Design review of the part built by this model. Coordinates are the model's own, in mm. Coordinates: 2 decimals unless noted, no trailing zeros. Loops run counter-clockwise (first coordinate to the right, second up) from the corner with the lowest first, then second, coordinate; pieces in that order, holes last. Notation, with made-up numbers: (-9, -15) - (39, -15) arc R25 ccw to (39, 4) - close; hole circle Ø9 at (-2, 6.5). An arc over 180 degrees is marked (long way). Use one line per item in the form item = value. Start each with the question number.
(1) Add section B-B (z = -54). State the section outline as (x, y) points.
(2) Add section A-A (z = -32.4). State the section outline as (x, y) points, plus the area to 3 significant figures.
(3) Clearance check with flat-ended pins moving along their axes: pin 1 Ø4.5 at (x, z) = (78.07, -32.4) entering from -Y; pin 2 Ø12.5 at (x, z) = (10, -10) entering from -Y. State where each tip first meets the part, or that it passes through.
(4) For L1, parallel to X at y = 2.75, z = -32.4; L2, parallel to Z at x = 140.5, y = 4.75; L3, parallel to X at y = 3, z = -10, list the stretches that pass through material, from the lowest coordinate up.
(5) Add section C-C (y = 2.25). Count the separate pieces of the cut face and the enclosed holes in it, plus the area to 3 significant figures.
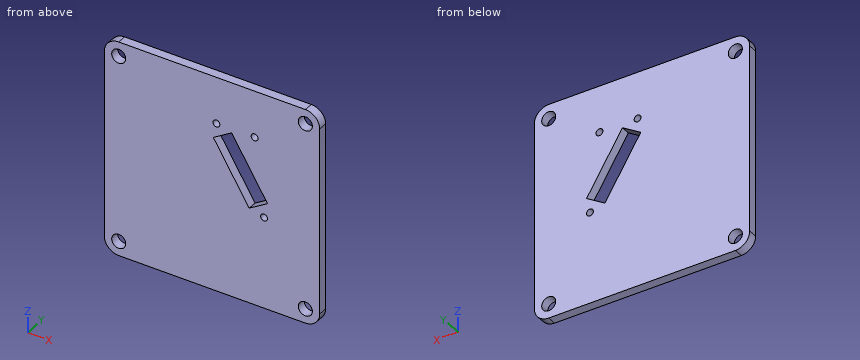
```python
from build123d import *

# Parameters (mm, degrees)
BOSS_EXTRUDE1_DEPTH = 6.35
SKETCH2_R           = 2.4
SKETCH2_R_2         = 4.9
CUT_EXTRUDE1_DEPTH  = 213.227054119


with BuildPart() as part:
    # Sketch1 → Boss-Extrude1 (new body)
    with BuildSketch(Plane(origin=(0, 0, 0), x_dir=(1, 0, 0), z_dir=(0, 1, 0))):
        with BuildLine():
            Line((10, 0), (140, 0))
            ThreePointArc((140, 0), (147.071067812, 2.928932188), (150, 10))
            Line((150, 10), (150, 140))
            ThreePointArc((150, 140), (147.071067812, 147.071067812), (140, 150))
            Line((140, 150), (10, 150))
            ThreePointArc((10, 150), (2.928932188, 147.071067812), (0, 140))
            Line((0, 140), (0, 10))
            ThreePointArc((0, 10), (2.928932188, 2.928932188), (10, 0))
        make_face()
    extrude(amount=BOSS_EXTRUDE1_DEPTH)

    # Sketch2 → Cut-Extrude1 (cut, through all)
    with BuildSketch(Plane(origin=(0, 6.35, 0), x_dir=(1, 0, 0), z_dir=(0, 1, 0))):
        with Locations(Location((78.068159546, 32.4, 0), (0, 0, 270))):
            Circle(SKETCH2_R)
        with Locations(Location((104.650093785, 32.4, 0), (0, 0, 270))):
            Circle(SKETCH2_R)
        with Locations(Location((111.276700611, 86.369381637, 0), (0, 0, 270))):
            Circle(SKETCH2_R)
        with Locations(Location((10, 140, 0), (0, 0, 270))):
            Circle(SKETCH2_R_2)
        with Locations(Location((10, 10, 0), (0, 0, 270))):
            Circle(SKETCH2_R_2)
        with Locations(Location((140, 140, 0), (0, 0, 270))):
            Circle(SKETCH2_R_2)
        with Locations(Location((140, 10, 0), (0, 0, 270))):
            Circle(SKETCH2_R_2)
        Polygon((75.891616838, 42.983313926), (88.666849341, 35.122433917), (113.627763661, 75.688055524), (100.852531159, 83.548935532), align=None)
    extrude(amount=-CUT_EXTRUDE1_DEPTH, mode=Mode.SUBTRACT)


solid = part.part
```
Computed values:
q1.outline = (0, 0) - (82.67, 0) - (82.67, 6.35) - (0, 6.35) - close; (100.28, 0) - (150, 0) - (150, 6.35) - (100.28, 6.35) - close
q2.outline = (0, 0) - (75.67, 0) - (75.67, 6.35) - (0, 6.35) - close; (80.47, 0) - (102.25, 0) - (102.25, 6.35) - (80.47, 6.35) - close; (107.05, 0) - (150, 0) - (150, 6.35) - (107.05, 6.35) - close
q2.area = 892 mm^2
q3.pin_1 = through
q3.pin_2 = 0
q4.L1 = 0 to 75.67, 80.47 to 102.25, 107.05 to 150
q4.L2 = -149.99 to -144.87, -135.13 to -14.87, -5.13 to -0.01
q4.L3 = 0 to 5.1, 14.9 to 135.1, 144.9 to 150
q5.separate_pieces = 1
q5.enclosed_holes = 8
q5.area = 21,300 mm^2
